CAD build for the part. Positions are in the model's coordinates, mm. A direction names the side the tool comes from. Round coordinates to 2 decimals unless told otherwise and drop trailing zeros. Write each loop counter-clockwise with the first axis right and the second up, starting at its lowest first coordinate (ties: lowest second). Pieces come first, ordered by that corner, then holes. Notation, with made-up numbers: (74.5, -32) -> (78.5, -32) arc R3 ccw to (78.5, -28) -> close; hole circle Ø11 at (51.5, -10.75). An arc over 180 degrees is marked (long way). Put each result on its own line as item: value. Start each with the question number.
1. Saw through at A-A on y = 0. List the corners of the cut face in (x, z), and give its area (3 significant figures).
2. Pull direction Y, two halves, no side cores. Call faces 1 (the cylindrical face through (-7.493, 0.33, 23.93)), 2 (the flat face through (4, -4, 23)), 3 (the flat face through (3, 0, 19)): pulls with the +Y half, pulls with the -Y half, needs draft (parallel to the pull), parting line crosses it, or undercut.
3. Flat gauge pins, fed straight in: P1, Ø3, axis at x = 4, z = 27.5, coming from the -Y side; P2, Ø5, axis at y = 2.5, z = 23, coming from the -X side; P3, Ø1, axis at x = 4, y = 4, coming from the -Z side. Where does each tip first touch, or does it go through?
4. Drill centre lines: line 1 (X direction, y = 4, z = 22.2); line 2 (Y direction, x = 0, z = 26.5). Where is each one in solid material? Low to high. Write a range as from..to.
5. Saw through at D-D on x = 4. List the corners of the cut face in (y, z).
6. 3-axis set-ups, long thin cutter, end or side, ignore diameter. For faces 4 (the cylindrical face through (-0.596, -2.685, 23.93)), 5 (the cylindrical face through (-5, -4, 21)): which of +Z, -Z, +X, -X, +Y, -Y reach the whole face in a straight line?
7. Saw through at C-C on z = 22. List the corners of the cut face in (x, y).
from build123d import *

# Parameters (mm, degrees)
CYLINDER1349_R     = 1
CYLINDER1349_DEPTH = 20
CYLINDER1351_R     = 1
CYLINDER1351_DEPTH = 20
CYLINDER1352_R     = 1
CYLINDER1352_DEPTH = 20
CYLINDER1345_R     = 1
CYLINDER1345_DEPTH = 20
TUBE120_R          = 7.5
TUBE120_R_2        = 2.75
TUBE120_DEPTH      = 10


with BuildPart() as obj1:
    # Cylinder1349 → Cylinder1349 (new body)
    with BuildSketch(Plane(origin=(4, -4, -88), x_dir=(0, 1, 0), z_dir=(0, 0, 1))):
        Circle(CYLINDER1349_R)
    extrude(amount=CYLINDER1349_DEPTH)


with BuildPart() as obj2:
    # Cylinder1351 → Cylinder1351 (new body)
    with BuildSketch(Plane(origin=(4, 4, -88), x_dir=(-1, 0, 0), z_dir=(0, 0, 1))):
        Circle(CYLINDER1351_R)
    extrude(amount=CYLINDER1351_DEPTH)


with BuildPart() as obj3:
    # Cylinder1352 → Cylinder1352 (new body)
    with BuildSketch(Plane(origin=(-4, 4, -88), x_dir=(0, -1, 0), z_dir=(0, 0, 1))):
        Circle(CYLINDER1352_R)
    extrude(amount=CYLINDER1352_DEPTH)


with BuildPart() as compound943:
    # Cylinder1345 → Cylinder1345 (new body)
    with BuildSketch(Plane(origin=(-4, -4, -88), x_dir=(1, 0, 0), z_dir=(0, 0, 1))):
        Circle(CYLINDER1345_R)
    extrude(amount=CYLINDER1345_DEPTH)

    # Compound943: union obj1, obj2, obj3
    add(obj1.part)
    add(obj2.part)
    add(obj3.part)


with BuildPart() as compound943_1:
    # Compound943 placement: moved
    add(compound943.part.moved(Location((0, 0, 91))))


with BuildPart() as cut484:
    # Tube120 → Tube120 (new body)
    with BuildSketch(Plane.XY.offset(19)):
        Circle(TUBE120_R)
        Circle(TUBE120_R_2, mode=Mode.SUBTRACT)
    extrude(amount=TUBE120_DEPTH)

    # Cut484: cut Compound943
    add(compound943_1.part, mode=Mode.SUBTRACT)


solid = cut484.part
Return value:
1. outline: (-7.5, 19) -> (-2.75, 19) -> (-2.75, 29) -> (-7.5, 29) -> close; (2.75, 19) -> (7.5, 19) -> (7.5, 29) -> (2.75, 29) -> close
1. area: 95.0 mm^2
2. face 1: parting line crosses it
2. face 2: undercut
2. face 3: needs draft
3. P1: stops at y = -7.07
3. P2: stops at x = -7.5
3. P3: stops at z = 23
4. line 1: x = -6.34..-5, -3..3, 5..6.34
4. line 2: y = -7.5..-2.75, 2.75..7.5
5. outline: (-6.34, 19) -> (-5, 19) -> (-5, 23) -> (-3, 23) -> (-3, 19) -> (3, 19) -> (3, 23) -> (5, 23) -> (5, 19) -> (6.34, 19) -> (6.34, 29) -> (-6.34, 29) -> close
6. face 4: +Z, -Z
6. face 5: -Z
7. outline: circle Ø15 at (0, 0); hole circle Ø2 at (-4, -4); hole circle Ø2 at (-4, 4); hole circle Ø5.5 at (0, 0); hole circle Ø2 at (4, -4); hole circle Ø2 at (4, 4)
